Here's the drawing with two shaded views (mm, measured from the low corner). I have some questions. Round coordinates to 2 decimals unless told otherwise and drop trailing zeros. Loops run counter-clockwise (first coordinate to the right, second up) from the corner with the lowest first, then second, coordinate; pieces in that order, holes last. Notation, with made-up numbers: (82, 72.5) - (117, 72.5) arc R5 ccw to (117, 81.5) - close; hole circle Ø5 at (-38, 65.25). An arc over 180 degrees is marked (long way). Use one line per item in the form item = value.
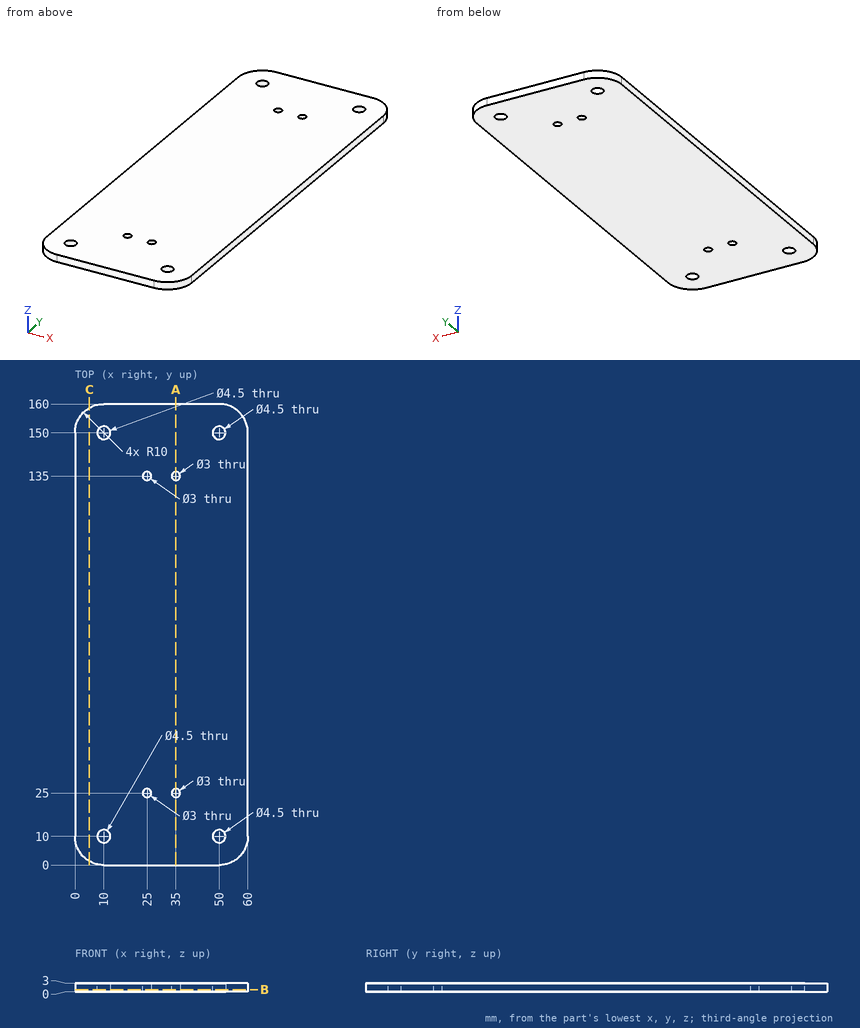
1. Please list where these lines run through material, in increasing order: line 1 along Y through (x, z) = (25, 0.75); line 2 along Y through (x, z) = (10, 1.85); line 3 along X through (y, z) = (8, 0.95).
Solution:
line_1 = 0 to 23.5, 26.5 to 133.5, 136.5 to 160
line_2 = 0 to 7.75, 12.25 to 147.75, 152.25 to 160
line_3 = 0.2 to 8.97, 11.03 to 48.97, 51.03 to 59.8
2. If we section it at B-B, the plane z = 0.7: Count the separate pieces of the cut face and the enclosed holes in it, plus the area to 3 significant figures.
Solution:
separate_pieces = 1
enclosed_holes = 8
area = 9,420 mm^2
3. If we section it at A-A, the plane x = 35: Write out the boundary of the cut face in (y, z).
Solution:
outline = (0, 0) - (23.5, 0) - (23.5, 3) - (0, 3) - close; (26.5, 0) - (133.5, 0) - (133.5, 3) - (26.5, 3) - close; (136.5, 0) - (160, 0) - (160, 3) - (136.5, 3) - close
4. If we section it at C-C, the plane x = 5: Write out the boundary of the cut face in (y, z), plus the area to 3 significant figures.
Solution:
outline = (1.34, 0) - (158.66, 0) - (158.66, 3) - (1.34, 3) - close
area = 472 mm^2
